Job drawing, mm, ordinate dimensions from the low corner. One solid piece. Give positions to 0.01 mm unless a question says otherwise; leave off trailing zeros. Loops run counter-clockwise (first coordinate to the right, second up) from the corner with the lowest first, then second, coordinate; pieces in that order, holes last. Notation, with made-up numbers: M -5,57.5 L 31,57.5 A25 cw 31,69.5 Z; hole C 0.5,76 d3. An arc over 180 degrees is marked long. One line per question, with ' | ' between items.
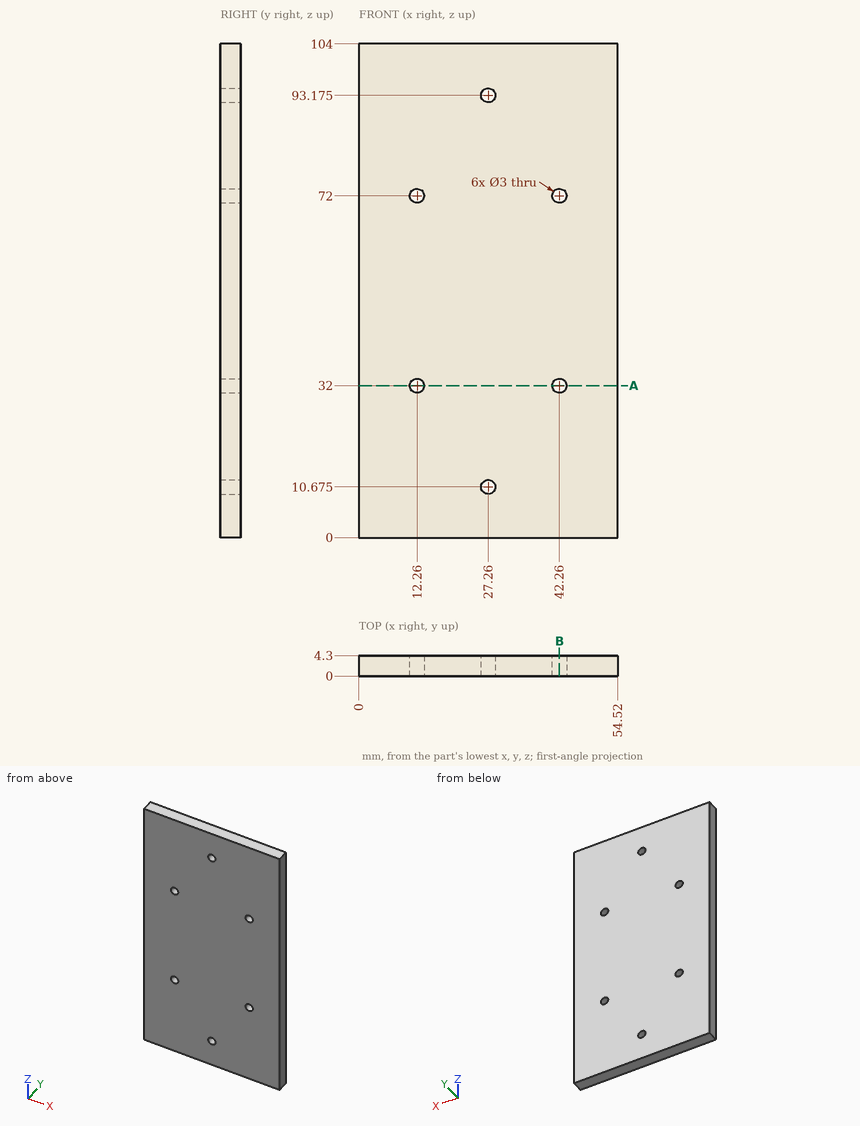
Item 1: Drill centre lines: line 1 along X through (y, z) = (1.45, 72); line 2 along Z through (x, y) = (42.26, 1.4). Where is each one in solid material? Low to high. Write a range as [from, to].
Conclusion:
line 1: [0, 10.76], [13.76, 40.76], [43.76, 54.52] | line 2: [0, 30.5], [33.5, 70.5], [73.5, 104]
Item 2: Saw through at B-B on x = 42.26. Give the cut face in (y, z), and give its area (3 significant figures).
Conclusion:
outline: M 0,0 L 4.3,0 L 4.3,30.5 L 0,30.5 Z; M 0,33.5 L 4.3,33.5 L 4.3,70.5 L 0,70.5 Z; M 0,73.5 L 4.3,73.5 L 4.3,104 L 0,104 Z | area: 421 mm²
Item 3: Saw through at A-A on z = 32. Give the cut face in (x, y).
Conclusion:
outline: M 0,0 L 10.76,0 L 10.76,4.3 L 0,4.3 Z; M 13.76,0 L 40.76,0 L 40.76,4.3 L 13.76,4.3 Z; M 43.76,0 L 54.52,0 L 54.52,4.3 L 43.76,4.3 Z
